Geometry check sheet. Reference: the model listing, model coordinates, mm. A direction names the side the tool comes from. Give positions to 0.01 mm unless a question says otherwise; leave off trailing zeros. Order: outer loops, then holes, each group sorted by start corner. A loop starts at its lowest first (then second) coordinate and runs counter-clockwise, first axis right, second up. Notation, with made-up numbers: M 22.5,17 L 79.5,17 A26 ccw 79.5,41 Z; hole C 53,52.25 d7. An arc over 180 degrees is marked long. Answer as CSV lines item,"result".
Autodesk Inventor part; units mm, degrees
ref_plane "Начальная плоскость" through (0, 0, 0) normal (0, 0, 1) x (1, 0, 0)
ref_plane "Конечная плоскость" through (0, 0, 210) normal (0, 0, 1) x (1, 0, 0)
ref_plane "YZ Plane" through (0, 0, 0) normal (1, 0, 0) x (0, 1, 0)
ref_plane "Начальная плоскость" through (0, 0, 0) normal (0, 0, 1) x (1, 0, 0)
ref_plane "Конечная плоскость" through (0, 0, 210) normal (0, 0, 1) x (1, 0, 0)
sketch "Эскиз" plane through (0, 0, 0) normal (0, 0, 1) x (1, 0, 0)
  line L0 (36, -32.5) -> (0, -32.5)
  line L1 (36, -32.5) -> (36, -28.696)
  line L2 (33.6994, -26.2039) -> (9.9215, -24.3017)
  line L3 (4.4, -18.3208) -> (4.4, 18.3208)
  line L4 (33.6994, 26.2039) -> (9.9215, 24.3017)
  line L5 (36, 28.696) -> (36, 32.5)
  line L6 (0, 32.5) -> (36, 32.5)
  line L7 (0, -32.5) -> (0, 32.5)
  arc A0 (4.4, -18.3208) -> (9.9215, -24.3017) centre (10.4, -18.3208) ccw
  arc A1 (9.9215, 24.3017) -> (4.4, 18.3208) centre (10.4, 18.3208) ccw
  arc A2 (36, -28.696) -> (33.6994, -26.2039) centre (33.5, -28.696) ccw
  arc A3 (33.6994, 26.2039) -> (36, 28.696) centre (33.5, 28.696) ccw
  line L8 (0, 45.5) -> (0, -45.5) construction
  line L9 (-7.2974, 0) -> (43.7847, 0) construction
  point P0 (36, -26.388)
  point P1 (4.4, -23.86)
  point P2 (4.4, 23.86)
  point P3 (36, 26.388)
  dimension "d3" = 36
  dimension "d5" = 4.4
  dimension "d7" = 65
  dimension "d9" = 8.64
  dimension "d11" = 8.64
  dimension "d13" = 6.112
  dimension "d15" = 6.112
  dimension "d22" = 6
  dimension "d23" = 2.5
  dimension "d24" = 32.5
  dimension "d25" = 0
extrude "Тело" add sketch "Эскиз" along normal up to surface (210 mm away) from surface at 0
sketch "Sketch3" plane through (0, 0, 0) normal (0, 0, 1) x (1, 0, 0)
  line L0 (0, 0) -> (10, 0)
ref_plane "Work Plane7" through (0, 0, 0) normal (0, -1, 0) x (1, 0, 0)
sketch "Sketch4" plane through (0, 0, 0) normal (0, -1, 0) x (1, 0, 0)
  line L0 (-2, 0) -> (12, 0)
  line L1 (-2, 210) -> (12, 210)
  dimension "d29" = 210
equation "\"d3\" = b"
equation "\"d7\" = ParH"
equation "\"d22\" = R"
equation "\"d23\" = R1"
equation "\"d24\" = 0.5 * d7"
equation "\"d16\" = G_L"
equation "\"R1\" = 2.5"
equation "\"R\" = 6"
equation "\"t1\" = 4.4"
equation "\"t2\" = 7.2"
equation "\"ParH\" = 65"
equation "\"b\" = 36"
equation "\"msp_x1\" = 0.04 * b"
equation "\"msp_x2\" = -0.08 * t1 + 0.04 * b"
equation "\"G_L\" = d29"
equation "\"ex\" = 0"
equation "\"G_OFFSET_START\" = 0"
equation "\"G_OFFSET_END\" = 0"
properties part number "Швеллер 6.5U-210 ГОСТ 8240-97"
(1) Gauge pin test, flat ends, axial feed: P1, Ø12, axis at y = 13.5, z = 28, coming from the -X side; P2, Ø5, axis at y = 4.5, z = 84, coming from the +X side. Record the tip position at first contact, or that the pin passes through.
The answers:
P1,"stops at x = 0"
P2,"stops at x = 4.4"
(2) Section check D-D on x = 22. Enter the section's corners in (y, z), then the cut area to 3 significant figures.
The answers:
outline,"M -32.5,0 L -25.27,0 L -25.27,210 L -32.5,210 Z; M 25.27,0 L 32.5,0 L 32.5,210 L 25.27,210 Z"
area,"3,040 mm2"
(3) Section check C-C on y = 6. Enter the section's corners in (x, z).
The answers:
outline,"M 0,0 L 4.4,0 L 4.4,210 L 0,210 Z"
(4) Section check A-A on z = 81.5. Enter the section's corners in (x, y), then the cut area to 3 significant figures.
The answers:
outline,"M 0,-32.5 L 36,-32.5 L 36,-28.7 A2.5 ccw 33.7,-26.2 L 9.92,-24.3 A6 cw 4.4,-18.32 L 4.4,18.32 A6 cw 9.92,24.3 L 33.7,26.2 A2.5 ccw 36,28.7 L 36,32.5 L 0,32.5 Z"
area,"763 mm2"
(5) Draft check along Y on faces 3 (the face through (4.4, 0, 104)), 4 (the face through (36, 31, 104)), 5 (the face through (18, -32.5, 104)). Enter one of: +Y half, -Y half, draft (parallel to the pull), parting line (faces both ways), or undercut.
The answers:
face 3,"undercut"
face 4,"draft"
face 5,"-Y half"
(6) Material ranges on line 1 (Y direction, x = 10, z = 151); line 2 (X direction, y = -10, z = 188.5); line 3 (Y direction, x = 7, z = 197), recorded low to high.
The answers:
line 1,"y = -32.5 to -24.31, 24.31 to 32.5"
line 2,"x = 0 to 4.4"
line 3,"y = -32.5 to -23.26, 23.26 to 32.5"
(7) Section check B-B on x = 13.5. Enter the section's corners in (y, z).
The answers:
outline,"M -32.5,0 L -24.59,0 L -24.59,210 L -32.5,210 Z; M 24.59,0 L 32.5,0 L 32.5,210 L 24.59,210 Z"
(8) Tool access check on faces 1 (the face through (3, 0, 210)), 2 (the face through (6, -22.4, 103.5)). Record the directions out of +Z, -Z, +X, -X, +Y, -Y that give a thin tool (end or side, any length) a straight path to the whole face; none if there is none.
The answers:
face 1,"+Z, +X, -X, +Y, -Y"
face 2,"+Z, -Z, +X"
